Geometry check sheet. Reference: the model listing, model coordinates, mm. Face numbers are marked on the shaded views. A direction names the side the tool comes from. Coordinates: 2 decimals unless noted, no trailing zeros. Loops run counter-clockwise (first coordinate to the right, second up) from the corner with the lowest first, then second, coordinate; pieces in that order, holes last. Notation, with made-up numbers: (77.25, 19) -> (99.25, 19) arc R27 ccw to (99.25, 51) -> close; hole circle Ø10 at (-18, 84.25). An arc over 180 degrees is marked (long way). Answer as a JSON object with one key per item and string values.
from build123d import *

# Parameters (mm, degrees)
F0_W     = 1117.6
F0_H     = 762
F0_W_2   = 338.666667
F0_H_2   = 336.55
F0_W_3   = 338.666666
F1_DEPTH = 381
F2_W     = 1117.6
F2_H     = 762
F3_DEPTH = 3.175


with BuildPart() as f1:
    # F0 (on Front) → F1 (new body)
    with BuildSketch(Plane.XZ):
        with Locations((558.8, -381)):
            Rectangle(F0_W, F0_H)
        with Locations((207.433334, -555.625)):
            Rectangle(F0_W_2, F0_H_2, mode=Mode.SUBTRACT)
        with Locations((558.8, -555.625)):
            Rectangle(F0_W_3, F0_H_2, mode=Mode.SUBTRACT)
        with Locations((910.166667, -555.625)):
            Rectangle(F0_W_2, F0_H_2, mode=Mode.SUBTRACT)
        with Locations((207.433334, -206.375)):
            Rectangle(F0_W_2, F0_H_2, mode=Mode.SUBTRACT)
        with Locations((558.8, -206.375)):
            Rectangle(F0_W_3, F0_H_2, mode=Mode.SUBTRACT)
        with Locations((910.166667, -206.375)):
            Rectangle(F0_W_2, F0_H_2, mode=Mode.SUBTRACT)
    extrude(amount=-F1_DEPTH)

    # F2 (on face) → F3 (join)
    with BuildSketch(Plane(origin=(0, 381, 0), x_dir=(-1, 0, 0), z_dir=(0, 1, 0))):
        with Locations((-558.8, -381)):
            Rectangle(F2_W, F2_H)
    extrude(amount=F3_DEPTH)


solid = f1.part
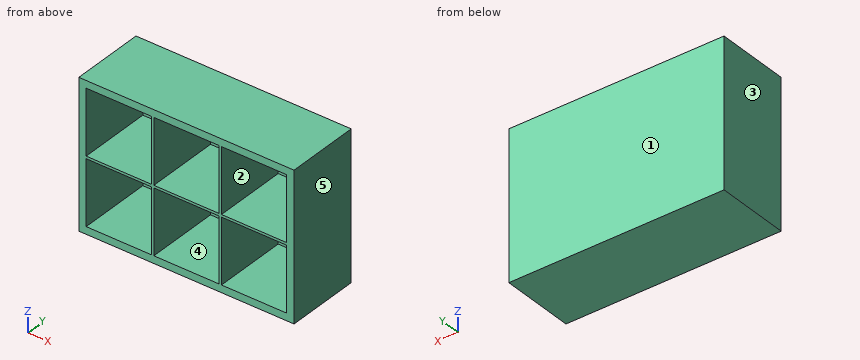
1. Section check C-C, the plane x = 248. Record the boundary of the cut face in (y, z) (3 decimals).
Evaluation:
{"outline": "(0, -762) -> (384.175, -762) -> (384.175, 0) -> (0, 0) -> (0, -38.1) -> (381, -38.1) -> (381, -374.65) -> (0, -374.65) -> (0, -387.35) -> (381, -387.35) -> (381, -723.9) -> (0, -723.9) -> close"}
2. Depth check by flat-ended pin: P1, Ø1.5, axis at x = 776.5, z = -646, coming from the -Y side. Enter the tip coordinate at first touch or a pass-through.
Evaluation:
{"P1": "stops at y = 381"}
3. Thickness scan on probe 1 along Z at (x, y) = (236, 248.5); probe 2 along X at (y, z) = (68.5, -626.5); probe 3 along Y at (x, z) = (176, -350) (3 decimals). Record the ranges inside material, lowest first. Write a range as from..to.
Evaluation:
{"probe 1": "z = -762..-723.9, -387.35..-374.65, -38.1..0", "probe 2": "x = 0..38.1, 376.77..389.47, 728.13..740.83, 1079.5..1117.6", "probe 3": "y = 381..384.175"}
4. Tool access check on the marked faces 1 and 2. Record the directions out of +Z, -Z, +X, -X, +Y, -Y that give a thin tool (end or side, any length) a straight path to the whole face; none if there is none.
Evaluation:
{"face 1": "+Z, -Z, +X, -X, +Y", "face 2": "-Y"}
5. Mould release check, pull along X, two halves, no side actions. Record for the marked faces 3, 4 and 5: released by +X, released by -X, zero draft, split by the parting line, or undercut.
Evaluation:
{"face 3": "released by -X", "face 4": "undercut", "face 5": "released by +X"}
6. Section check A-A, the plane y = 334. Record the boundary of the cut face in (x, z), then the cut area to 3 significant figures.
Evaluation:
{"outline": "(0, -762) -> (1117.6, -762) -> (1117.6, 0) -> (0, 0) -> close; hole (38.1, -723.9) -> (376.77, -723.9) -> (376.77, -387.35) -> (38.1, -387.35) -> close; hole (38.1, -374.65) -> (376.77, -374.65) -> (376.77, -38.1) -> (38.1, -38.1) -> close; hole (389.47, -723.9) -> (728.13, -723.9) -> (728.13, -387.35) -> (389.47, -387.35) -> close; hole (389.47, -374.65) -> (728.13, -374.65) -> (728.13, -38.1) -> (389.47, -38.1) -> close; hole (740.83, -723.9) -> (1079.5, -723.9) -> (1079.5, -387.35) -> (740.83, -387.35) -> close; hole (740.83, -374.65) -> (1079.5, -374.65) -> (1079.5, -38.1) -> (740.83, -38.1) -> close", "area": "168,000 mm^2"}
7. Section check B-B, the plane z = -506.5. Record the boundary of the cut face in (x, y) (3 decimals), then the cut area to 3 significant figures.
Evaluation:
{"outline": "(0, 0) -> (38.1, 0) -> (38.1, 381) -> (376.767, 381) -> (376.767, 0) -> (389.467, 0) -> (389.467, 381) -> (728.133, 381) -> (728.133, 0) -> (740.833, 0) -> (740.833, 381) -> (1079.5, 381) -> (1079.5, 0) -> (1117.6, 0) -> (1117.6, 384.175) -> (0, 384.175) -> close", "area": "42,300 mm^2"}
